Part model, mm, in its own coordinate system. A direction names the side the tool comes from. Give positions to 0.01 mm unless a question says otherwise; leave off trailing zeros. Loops run counter-clockwise (first coordinate to the right, second up) from the corner with the lowest first, then second, coordinate; pieces in that order, holes last. Notation, with made-up numbers: M 75,24 L 124,24 A21 ccw 124,43 Z; hole C -35.5,-12.75 d10. An arc over 180 degrees is marked long. Answer in a Markdown table with one row per item.
from build123d import *

# Parameters (mm, degrees)
SKETCH_1_W          = 42
SKETCH_1_H          = 42
EXTRUDE_1_DEPTH     = 60
SKETCH_2_R          = 1.5
CUT_EXTRUDE_1_DEPTH = 65
SKETCH_3_R          = 11
EXTRUDE_2_DEPTH     = 2
SKETCH_4_R          = 2.5
EXTRUDE_3_DEPTH     = 22
CHAMFER_1_SIZE      = 0.3
CHAMFER_2_SIZE      = 4
CUT_EXTRUDE_2_DEPTH = 39


with BuildPart() as part:
    # Эскиз1 → Бобышка-Вытянуть1 (new body)
    with BuildSketch(Plane.XY):
        with Locations((-12.492530381, 4.702380952)):
            Rectangle(SKETCH_1_W, SKETCH_1_H)
    extrude(amount=EXTRUDE_1_DEPTH)

    # Эскиз2 → Вырез-Вытянуть1 (cut)
    with BuildSketch(Plane(origin=(0, 0, 0), x_dir=(-1, 0, 0), z_dir=(0, 0, -1))):
        with Locations((-3.007469619, 20.202380952)):
            Circle(SKETCH_2_R)
        with Locations((27.992530381, 20.202380952)):
            Circle(SKETCH_2_R)
        with Locations((27.992530381, -10.797619048)):
            Circle(SKETCH_2_R)
        with Locations((-3.007469619, -10.797619048)):
            Circle(SKETCH_2_R)
    extrude(amount=-CUT_EXTRUDE_1_DEPTH, mode=Mode.SUBTRACT)

    # Эскиз3 → Бобышка-Вытянуть2 (add)
    with BuildSketch(Plane(origin=(0, 0, 0), x_dir=(-1, 0, 0), z_dir=(0, 0, -1))):
        with Locations(Location((12.492530381, 4.702380952, 0), (0, 0, 180))):
            Circle(SKETCH_3_R)
    extrude(amount=EXTRUDE_2_DEPTH)

    # Эскиз4 → Бобышка-Вытянуть3 (add)
    with BuildSketch(Plane(origin=(0, 0, -2), x_dir=(-1, 0, 0), z_dir=(0, 0, -1))):
        with Locations((12.492530381, 4.702380952)):
            Circle(SKETCH_4_R)
    extrude(amount=EXTRUDE_3_DEPTH)

    # Фаска1
    chamfer_1_edges = [part.edges().sort_by_distance(p)[0] for p in [
        (-9.992530381, 4.702380952, -24),
    ]]
    chamfer(chamfer_1_edges, length=CHAMFER_1_SIZE)

    # Фаска2
    chamfer_2_edges = [part.edges().sort_by_distance(p)[0] for p in [
        (-33.492530381, 25.702380952, 30),
        (8.507469619, 25.702380952, 30),
        (8.507469619, -16.297619048, 30),
        (-33.492530381, -16.297619048, 30),
    ]]
    chamfer(chamfer_2_edges, length=CHAMFER_2_SIZE)

    # Эскиз5 → Вырез-Вытянуть2 (cut)
    with BuildSketch(Plane(origin=(0, 0, 11), x_dir=(-1, 0, 0), z_dir=(0, 0, -1))):
        Polygon((-8.507469619, 18.873953828), (-1.679042494, 25.702380952), (-4.507469619, 25.702380952), (-8.507469619, 21.702380952), align=None)
        Polygon((-8.507469619, -9.469191923), (-8.507469619, -12.297619048), (-4.507469619, -16.297619048), (-1.679042494, -16.297619048), align=None)
        Polygon((26.664103256, 25.702380952), (33.492530381, 18.873953828), (33.492530381, 21.702380952), (29.492530381, 25.702380952), align=None)
        Polygon((33.492530381, -9.469191923), (26.664103256, -16.297619048), (29.492530381, -16.297619048), (33.492530381, -12.297619048), align=None)
    extrude(amount=-CUT_EXTRUDE_2_DEPTH, mode=Mode.SUBTRACT)


solid = part.part
(1) Saw through at A-A (x = -28). Write the cut outline in (y, z), plus the area to 3 significant figures.
Recorded:
| item | result |
|---|---|
| outline | M -16.3,0 L -12.3,0 L -12.3,60 L -16.3,60 L -16.3,50 L -14.96,50 L -14.96,11 L -16.3,11 Z; M -9.3,0 L 18.7,0 L 18.7,60 L -9.3,60 Z; M 21.7,0 L 25.7,0 L 25.7,11 L 24.37,11 L 24.37,50 L 25.7,50 L 25.7,60 L 21.7,60 Z |
| area | 2,060 mm^2 |
(2) Saw through at D-D (x = -9). Write the cut outline in (y, z), plus the area to 3 significant figures.
Recorded:
| item | result |
|---|---|
| outline | M -16.3,0 L -5.73,0 L -5.73,-2 L 15.13,-2 L 15.13,0 L 25.7,0 L 25.7,60 L -16.3,60 Z |
| area | 2,560 mm^2 |
(3) Saw through at B-B (z = 8). Write the cut outline in (x, y), plus the area to 3 significant figures.
Recorded:
| item | result |
|---|---|
| outline | M -33.49,-12.3 L -29.49,-16.3 L 4.51,-16.3 L 8.51,-12.3 L 8.51,21.7 L 4.51,25.7 L -29.49,25.7 L -33.49,21.7 Z; hole C -27.99,-10.8 d3; hole C -27.99,20.2 d3; hole C 3.01,-10.8 d3; hole C 3.01,20.2 d3 |
| area | 1,700 mm^2 |
(4) Pin check, flat tips, straight feed: pin 1 Ø2.5 at (x, y) = (3.01, 20.2) entering from +Z; pin 2 Ø2 at (x, y) = (-29.5, 21.5) entering from -Z; pin 3 Ø12.5 at (x, y) = (-21, 1) entering from -Z. Stop position of each tip, or through.
Recorded:
| item | result |
|---|---|
| pin 1 | passes through |
| pin 2 | stops at z = 0 |
| pin 3 | stops at z = -2 |
(5) Which spindle directions (+Z, -Z, +X, -X, +Y, -Y) get a long thin tool onto all of the face, cutting with end or side? Do faces 1 (the face through (-31, -14, 50)), 2 (the face through (-31.465, 23.73, 5.423)), 3 (the face through (6, -13, 11)), 4 (the face through (-2, 1.4, -1)), 5 (the face through (6, 23, 50)). Say none if no direction does.
Recorded:
| item | result |
|---|---|
| face 1 | -X, -Y |
| face 2 | +Z, -Z, -X, +Y |
| face 3 | +X, -Y |
| face 4 | -Z |
| face 5 | +X, +Y |
(6) Drill centre lines: line 1 along Y through (x, z) = (-28, 22); line 2 along Z through (x, y) = (-0.5, -9); line 3 along Z through (x, y) = (-10.5, 10). Where is each one in solid material? Low to high.
Recorded:
| item | result |
|---|---|
| line 1 | y = -14.96 to -12.3, -9.3 to 18.7, 21.7 to 24.37 |
| line 2 | z = 0 to 60 |
| line 3 | z = -2 to 60 |
(7) Saw through at C-C (y = 13). Write the cut outline in (x, z).
Recorded:
| item | result |
|---|---|
| outline | M -33.49,0 L -19.71,0 L -19.71,-2 L -5.27,-2 L -5.27,0 L 8.51,0 L 8.51,60 L -33.49,60 Z |
(8) Pull direction Z, two halves, no side cores. Call faces 6 (the face through (6, -13, 50)), 7 (the face through (-13, 5, 60)), 8 (the face through (6.54, 23.67, 5.42)): +Z half, -Z half, draft (parallel to the pull), parting line (faces both ways), or undercut.
Recorded:
| item | result |
|---|---|
| face 6 | undercut |
| face 7 | +Z half |
| face 8 | draft |
